```python
from build123d import *

# Parameters (mm, degrees)
F0_W     = 151.13
F0_H     = 35.306
F1_DEPTH = 1.778
F2_W     = 151.13
F2_H     = 35.306
F4_DEPTH = 1.778
F3_W     = 8.89
F3_H     = 6.096
F3_W_2   = 9.525
F3_H_2   = 14.478
F5_DEPTH = 2.54


with BuildPart() as f1:
    # F0 (on Top) → F1 (new body)
    with BuildSketch(Plane.XY):
        with Locations((-0.822666, -120.916817)):
            Rectangle(F0_W, F0_H)
    extrude(amount=F1_DEPTH)


with BuildPart() as f4:
    # F2 (on Top) → F4 (new body)
    with BuildSketch(Plane.XY):
        Rectangle(F2_W, F2_H)
    extrude(amount=F4_DEPTH)

    # F3 (on face) → F5 (cut)
    with BuildSketch(Plane.XY):
        with Locations((-3.99227, -9.652)):
            Rectangle(F3_W, F3_H)
        with Locations((-20.438026, -9.652)):
            Rectangle(F3_W, F3_H)
        with Locations((9.91423, -5.461)):
            Rectangle(F3_W_2, F3_H_2)
    extrude(amount=F5_DEPTH, mode=Mode.SUBTRACT)


solid = f4.part
```
Can you work these out from the model? Positions are in its coordinate system, mm. Give positions to 0.01 mm unless a question says otherwise; leave off trailing zeros. Loops run counter-clockwise (first coordinate to the right, second up) from the corner with the lowest first, then second, coordinate; pieces in that order, holes last. Notation, with made-up numbers: M -37,-25.75 L 3,-25.75 A10 cw 3,-21.75 Z; hole C 36.25,14 d2. An arc over 180 degrees is marked long. One line per question, with ' | ' between items. Start each with the question number.
Q1. If we section it at C-C (z = 0.95): Please give me the cut outline in (x, y) (3 decimals), plus the area to 3 significant figures.
Q2. If we section it at B-B (y = -1.5): Please give me the cut outline in (x, z) (3 decimals), plus the area to 3 significant figures.
Q3. If we section it at A-A (x = 11): Please give me the cut outline in (y, z), plus the area to 3 significant figures.
Q4. If I drill on line 1 (Y direction, x = -22.5, z = 1.6); line 2 (X direction, y = -6, z = 1.3) (3 decimals); line 3 (Y direction, x = 5.5, z = 0.85), over which ranges is the centre line in solid material (lowest first)? Write a range as from..to.
Q5. If we mould it in two halves opening along Z, with no side actions, what happens to faces 1 (the flat face through (-1, 0, 0)), 2 (the flat face through (-1, 0, 1.778))? For each: +Z half, -Z half, draft (parallel to the pull), parting line (faces both ways), or undercut.
Computed:
1) outline: M -75.565,-17.653 L 75.565,-17.653 L 75.565,17.653 L -75.565,17.653 Z; hole M -24.883,-12.7 L -15.993,-12.7 L -15.993,-6.604 L -24.883,-6.604 Z; hole M -8.437,-12.7 L 0.453,-12.7 L 0.453,-6.604 L -8.437,-6.604 Z; hole M 5.152,-12.7 L 14.677,-12.7 L 14.677,1.778 L 5.152,1.778 Z | area: 5,090 mm²
2) outline: M -75.565,0 L 5.152,0 L 5.152,1.778 L -75.565,1.778 Z; M 14.677,0 L 75.565,0 L 75.565,1.778 L 14.677,1.778 Z | area: 252 mm²
3) outline: M -17.65,0 L -12.7,0 L -12.7,1.78 L -17.65,1.78 Z; M 1.78,0 L 17.65,0 L 17.65,1.78 L 1.78,1.78 Z | area: 37.0 mm²
4) line 1: y = -17.65..-12.7, -6.6..17.65 | line 2: x = -75.565..5.152, 14.677..75.565 | line 3: y = -17.65..-12.7, 1.78..17.65
5) face 1: -Z half | face 2: +Z half
